Autodesk Fusion 360 part; units mm, degrees
sketch "Sketch1" plane through (0, 12, 0) normal (0, -1, 0) x (1, 0, 0)
  line L0 (-41.8393, 72.4678) -> (-83.6786, 0)
  line L1 (-83.6786, 0) -> (-41.8393, -72.4678)
  line L2 (-41.8393, -72.4678) -> (41.8393, -72.4678)
  line L3 (41.8393, -72.4678) -> (83.6786, 0)
  line L4 (83.6786, 0) -> (41.8393, 72.4678)
  line L5 (41.8393, 72.4678) -> (-41.8393, 72.4678)
  line L6 (-41.8393, 72.4678) -> (41.8393, 72.4678)
  line L7 (41.8393, 72.4678) -> (83.6786, 0)
  line L8 (83.6786, 0) -> (41.8393, -72.4678)
  line L9 (41.8393, -72.4678) -> (-41.8393, -72.4678)
  line L10 (-41.8393, -72.4678) -> (-83.6786, 0)
  line L11 (-83.6786, 0) -> (-41.8393, 72.4678)
  line L12 (82.0621, 0) -> (41.031, -71.0678)
  line L13 (41.031, -71.0678) -> (-41.031, -71.0678)
  line L14 (-41.031, -71.0678) -> (-82.0621, 0)
  line L15 (-82.0621, 0) -> (-41.031, 71.0678)
  line L16 (-41.031, 71.0678) -> (41.031, 71.0678)
  line L17 (41.031, 71.0678) -> (82.0621, 0)
  dimension "d1" = 1.4
sketch "Sketch2" plane through (0, 12, 0) normal (0, 1, 0) x (-1, 0, 0)
  line L0 (-42.4167, 73.4678) -> (42.4167, 73.4678)
  line L1 (42.4167, 73.4678) -> (84.8333, 0)
  line L2 (84.8333, 0) -> (42.4167, -73.4678)
  line L3 (42.4167, -73.4678) -> (-42.4167, -73.4678)
  line L4 (-42.4167, -73.4678) -> (-84.8333, 0)
  line L5 (-84.8333, 0) -> (-42.4167, 73.4678)
  line L6 (-43.5714, 75.4678) -> (-87.1427, 0)
  line L7 (-87.1427, 0) -> (-43.5714, -75.4678)
  line L8 (-43.5714, -75.4678) -> (43.5714, -75.4678)
  line L9 (43.5714, -75.4678) -> (87.1427, 0)
  line L10 (87.1427, 0) -> (43.5714, 75.4678)
  line L11 (43.5714, 75.4678) -> (-43.5714, 75.4678)
  line L12 (-43.5714, 75.4678) -> (43.5714, 75.4678)
  line L13 (87.1427, 0) -> (43.5714, 75.4678)
  line L14 (87.1427, 0) -> (43.5714, -75.4678)
  line L15 (43.5714, -75.4678) -> (-43.5714, -75.4678)
  line L16 (-43.5714, -75.4678) -> (-87.1427, 0)
  line L17 (-87.1427, 0) -> (-43.5714, 75.4678)
sketch "Sketch3" plane through (0, 4, 0) normal (0, 1, 0) x (-1, 0, 0)
  line L0 (-38.9526, -67.4678) -> (-77.9051, 0)
  line L1 (-77.9051, 0) -> (-38.9526, 67.4678)
  line L2 (-38.9526, 67.4678) -> (38.9526, 67.4678)
  line L3 (38.9526, 67.4678) -> (77.9051, 0)
  line L4 (77.9051, 0) -> (38.9526, -67.4678)
  line L5 (38.9526, -67.4678) -> (-38.9526, -67.4678)
  line L6 (-84.8333, 0) -> (-42.4167, -73.4678)
  line L7 (-42.4167, -73.4678) -> (42.4167, -73.4678)
  line L8 (42.4167, -73.4678) -> (84.8333, 0)
  line L9 (84.8333, 0) -> (42.4167, 73.4678)
  line L10 (42.4167, 73.4678) -> (-42.4167, 73.4678)
  line L11 (-42.4167, 73.4678) -> (-84.8333, 0)
  line L12 (42.4167, -73.4678) -> (84.8333, 0)
  line L13 (42.4167, 73.4678) -> (84.8333, 0)
  line L14 (42.4167, 73.4678) -> (-42.4167, 73.4678)
  line L15 (-42.4167, 73.4678) -> (-84.8333, 0)
  line L16 (-84.8333, 0) -> (-42.4167, -73.4678)
  line L17 (-42.4167, -73.4678) -> (42.4167, -73.4678)
  line L18 (-42.4167, 73.4678) -> (-84.8333, 0)
  line L19 (-41.8393, -72.4678) -> (41.8393, -72.4678)
  line L20 (41.8393, -72.4678) -> (83.6786, 0)
  line L21 (41.8393, 72.4678) -> (83.6786, 0)
  line L22 (41.8393, 72.4678) -> (-41.8393, 72.4678)
  line L23 (-41.8393, 72.4678) -> (-83.6786, 0)
  line L24 (-83.6786, 0) -> (-41.8393, -72.4678)
  line L25 (41.031, 71.0678) -> (-41.031, 71.0678)
  line L26 (-41.031, 71.0678) -> (-82.0621, 0)
  line L27 (-82.0621, 0) -> (-41.031, -71.0678)
  line L28 (-41.031, -71.0678) -> (41.031, -71.0678)
  line L29 (41.031, -71.0678) -> (82.0621, 0)
  line L30 (41.031, 71.0678) -> (82.0621, 0)
  dimension "d2" = -1
  dimension "d3" = -2.4
sketch "Sketch4" plane through (0, 13, 0) normal (0, -1, 0) x (1, 0, 0)
  arc A0 (44.7261, 67.4678) -> (36.0658, 72.4678) centre (36.0658, 62.4678) ccw
  line L0 (44.7261, 67.4678) -> (80.7919, 5)
  arc A1 (80.7919, -5) -> (80.7919, 5) centre (72.1316, 0) ccw
  line L1 (80.7919, -5) -> (44.7261, -67.4678)
  arc A2 (36.0658, -72.4678) -> (44.7261, -67.4678) centre (36.0658, -62.4678) ccw
  line L2 (36.0658, -72.4678) -> (-36.0658, -72.4678)
  arc A3 (-44.7261, -67.4678) -> (-36.0658, -72.4678) centre (-36.0658, -62.4678) ccw
  line L3 (-44.7261, -67.4678) -> (-80.7919, -5)
  arc A4 (-80.7919, 5) -> (-80.7919, -5) centre (-72.1316, 0) ccw
  line L4 (-80.7919, 5) -> (-44.7261, 67.4678)
  arc A5 (-36.0658, 72.4678) -> (-44.7261, 67.4678) centre (-36.0658, 62.4678) ccw
  line L5 (-36.0658, 72.4678) -> (36.0658, 72.4678)
  line L6 (42.4167, 73.4678) -> (-42.4167, 73.4678)
  line L7 (-42.4167, 73.4678) -> (-84.8333, 0)
  line L8 (-84.8333, 0) -> (-42.4167, -73.4678)
  line L9 (-42.4167, -73.4678) -> (42.4167, -73.4678)
  line L10 (42.4167, -73.4678) -> (84.8333, 0)
  line L11 (84.8333, 0) -> (42.4167, 73.4678)
  line L12 (-42.4167, 73.4678) -> (-32.4167, 73.4678)
  line L13 (-42.4167, 73.4678) -> (-47.4167, 64.8076)
  line L14 (-32.4167, 73.4678) -> (-32.4167, 56.1473)
  line L15 (-47.4167, 64.8076) -> (-32.4167, 56.1473)
  dimension "d4" = 10
  dimension "d5" = 0
extrude "Extrude1" add sketch "Sketch2" along normal blind 3 contours L0 L1 L2 L3 L4 L5 | L6 L7 L8 L9 L10 L11 L12 L13 L14 L15 L16 L17
extrude "Extrude2" cut sketch "Sketch3" along normal blind -1 and the other way blind -9 contours L6 L7 L8 L9 L10 L11 L12 L13 L14 L15 L16 L17 L18
move_face "OffsetFaces1" [suppressed]
extrude "Extrude3" cut sketch "Sketch1" against normal blind 2.6 contours L12 L13 L14 L15 L16 L17
fillet "Fillet1" radius 10 6 edges at (-83.6786, 12.5, 0) (-41.8393, 12.5, 72.4678) (41.8393, 12.5, 72.4678) (83.6786, 12.5, 0) (41.8393, 12.5, -72.4678) (-41.8393, 12.5, -72.4678)
fillet "Fillet1" radius 10 6 edges at (-41.031, 13.3, 71.0678) (-82.0621, 13.3, 0) (-41.031, 13.3, -71.0678) (41.031, 13.3, -71.0678) (82.0621, 13.3, 0) (41.031, 13.3, 71.0678)
chamfer "Chamfer1" distance 1 angle 45 18 edges at (63.625, 12, 36.7339) (63.625, 12, -36.7339) (82.1316, 12, 0) (62.759, 12, -36.2339) (41.0658, 12, -71.1281) (0, 12, -72.4678) (-41.0658, 12, -71.1281) (-62.759, 12, -36.2339) (-82.1316, 12, 0) (-62.759, 12, 36.2339) (-41.0658, 12, 71.1281) (0, 12, 72.4678) (41.0658, 12, 71.1281) (62.759, 12, 36.2339) (0, 12, 73.4678) (-63.625, 12, 36.7339) (-63.625, 12, -36.7339) (0, 12, -73.4678)
sketch "Sketch5" plane through (0, 14.6, 0) normal (0, -1, 0) x (1, 0, 0)
  arc A0 (43.9178, 66.0678) -> (35.2575, 71.0678) centre (35.2575, 61.0678) ccw
  line L0 (35.2575, 71.0678) -> (-35.2575, 71.0678)
  arc A1 (-35.2575, 71.0678) -> (-43.9178, 66.0678) centre (-35.2575, 61.0678) ccw
  line L1 (-43.9178, 66.0678) -> (-79.1753, 5)
  arc A2 (-79.1753, 5) -> (-79.1753, -5) centre (-70.515, 0) ccw
  line L2 (-79.1753, -5) -> (-43.9178, -66.0678)
  arc A3 (-43.9178, -66.0678) -> (-35.2575, -71.0678) centre (-35.2575, -61.0678) ccw
  line L3 (-35.2575, -71.0678) -> (35.2575, -71.0678)
  arc A4 (35.2575, -71.0678) -> (43.9178, -66.0678) centre (35.2575, -61.0678) ccw
  line L4 (43.9178, -66.0678) -> (79.1753, -5)
  arc A5 (79.1753, -5) -> (79.1753, 5) centre (70.515, 0) ccw
  line L5 (79.1753, 5) -> (43.9178, 66.0678)
  line L6 (0, 0) -> (-80.515, 0)
  line L7 (-40.2575, 69.7281) -> (0, 0)
  line L8 (40.2575, 69.7281) -> (-40.2575, -69.7281)
  line L9 (40.2575, -69.7281) -> (0, 0)
  line L10 (80.515, 0) -> (0, 0)
extrude "Extrude11" add 1 faces at (2.8868, 14.6, -1.6667) along direction (0, -1, 0) blind 3
extrude "Extrude5" [suppressed]
extrude "Extrude6" [suppressed]
extrude "Extrude7" [suppressed]
extrude "Extrude8" [suppressed]
extrude "Extrude9" [suppressed]
sketch "Sketch6" plane through (0, 12, 0) normal (0, -1, 0) x (1, 0, 0)
  line L0 (-35.2575, 71.0678) -> (35.2575, 71.0678)
  arc A0 (43.9178, 66.0678) -> (35.2575, 71.0678) centre (35.2575, 61.0678) ccw
  line L1 (43.9178, 66.0678) -> (79.1753, 5)
  arc A1 (79.1753, -5) -> (79.1753, 5) centre (70.515, 0) ccw
  line L2 (79.1753, -5) -> (43.9178, -66.0678)
  arc A2 (35.2575, -71.0678) -> (43.9178, -66.0678) centre (35.2575, -61.0678) ccw
  line L3 (35.2575, -71.0678) -> (-35.2575, -71.0678)
  arc A3 (-43.9178, -66.0678) -> (-35.2575, -71.0678) centre (-35.2575, -61.0678) ccw
  line L4 (-43.9178, -66.0678) -> (-79.1753, -5)
  arc A4 (-79.1753, 5) -> (-79.1753, -5) centre (-70.515, 0) ccw
  line L5 (-79.1753, 5) -> (-43.9178, 66.0678)
  line L6 (-43.86, 66.9678) -> (-79.9259, 4.5)
  arc A5 (-79.9259, 4.5) -> (-79.9259, -4.5) centre (-72.1316, 0) ccw
  line L7 (-79.9259, -4.5) -> (-43.86, -66.9678)
  arc A6 (-43.86, -66.9678) -> (-36.0658, -71.4678) centre (-36.0658, -62.4678) ccw
  line L8 (-36.0658, -71.4678) -> (36.0658, -71.4678)
  arc A7 (36.0658, -71.4678) -> (43.86, -66.9678) centre (36.0658, -62.4678) ccw
  line L9 (43.86, -66.9678) -> (79.9259, -4.5)
  arc A8 (79.9259, -4.5) -> (79.9259, 4.5) centre (72.1316, 0) ccw
  line L10 (79.9259, 4.5) -> (43.86, 66.9678)
  arc A9 (43.86, 66.9678) -> (36.0658, 71.4678) centre (36.0658, 62.4678) ccw
  line L11 (36.0658, 71.4678) -> (-36.0658, 71.4678)
  arc A10 (-35.2575, 71.0678) -> (-43.9178, 66.0678) centre (-35.2575, 61.0678) ccw
  arc A11 (-36.0658, 71.4678) -> (-43.86, 66.9678) centre (-36.0658, 62.4678) ccw
  line L12 (-79.1753, 5) -> (-43.9178, 66.0678)
  arc A12 (-35.2575, 71.0678) -> (-43.9178, 66.0678) centre (-35.2575, 61.0678) ccw
  line L13 (-35.2575, 71.0678) -> (35.2575, 71.0678)
  arc A13 (43.9178, 66.0678) -> (35.2575, 71.0678) centre (35.2575, 61.0678) ccw
  line L14 (43.9178, 66.0678) -> (79.1753, 5)
  arc A14 (79.1753, -5) -> (79.1753, 5) centre (70.515, 0) ccw
  line L15 (79.1753, -5) -> (43.9178, -66.0678)
  arc A15 (35.2575, -71.0678) -> (43.9178, -66.0678) centre (35.2575, -61.0678) ccw
  line L16 (35.2575, -71.0678) -> (-35.2575, -71.0678)
  arc A16 (-43.9178, -66.0678) -> (-35.2575, -71.0678) centre (-35.2575, -61.0678) ccw
  line L17 (-43.9178, -66.0678) -> (-79.1753, -5)
  arc A17 (-79.1753, 5) -> (-79.1753, -5) centre (-70.515, 0) ccw
  arc A18 (79.9259, -4.5) -> (79.9259, 4.5) centre (72.1316, 0) ccw
  line L18 (79.9259, 4.5) -> (43.86, 66.9678)
  arc A19 (43.86, 66.9678) -> (36.0658, 71.4678) centre (36.0658, 62.4678) ccw
  line L19 (36.0658, 71.4678) -> (-36.0658, 71.4678)
  arc A20 (-36.0658, 71.4678) -> (-43.86, 66.9678) centre (-36.0658, 62.4678) ccw
  line L20 (-43.86, 66.9678) -> (-79.9259, 4.5)
  arc A21 (-79.9259, 4.5) -> (-79.9259, -4.5) centre (-72.1316, 0) ccw
  line L21 (-79.9259, -4.5) -> (-43.86, -66.9678)
  arc A22 (-43.86, -66.9678) -> (-36.0658, -71.4678) centre (-36.0658, -62.4678) ccw
  line L22 (-36.0658, -71.4678) -> (36.0658, -71.4678)
  arc A23 (36.0658, -71.4678) -> (43.86, -66.9678) centre (36.0658, -62.4678) ccw
  line L23 (43.86, -66.9678) -> (79.9259, -4.5)
  arc A24 (42.8785, 65.4678) -> (35.2575, 69.8678) centre (35.2575, 61.0678) ccw
  line L24 (-35.2575, 69.8678) -> (35.2575, 69.8678)
  arc A25 (-35.2575, 69.8678) -> (-42.8785, 65.4678) centre (-35.2575, 61.0678) ccw
  line L25 (-78.1361, 4.4) -> (-42.8785, 65.4678)
  arc A26 (-78.1361, 4.4) -> (-78.1361, -4.4) centre (-70.515, 0) ccw
  line L26 (-42.8785, -65.4678) -> (-78.1361, -4.4)
  arc A27 (-42.8785, -65.4678) -> (-35.2575, -69.8678) centre (-35.2575, -61.0678) ccw
  line L27 (35.2575, -69.8678) -> (-35.2575, -69.8678)
  arc A28 (35.2575, -69.8678) -> (42.8785, -65.4678) centre (35.2575, -61.0678) ccw
  line L28 (78.1361, -4.4) -> (42.8785, -65.4678)
  arc A29 (78.1361, -4.4) -> (78.1361, 4.4) centre (70.515, 0) ccw
  line L29 (42.8785, 65.4678) -> (78.1361, 4.4)
  arc A30 (-35.2575, 70.0678) -> (-43.0518, 65.5678) centre (-35.2575, 61.0678) ccw
  line L30 (-78.3093, 4.5) -> (-43.0518, 65.5678)
  arc A31 (-78.3093, 4.5) -> (-78.3093, -4.5) centre (-70.515, 0) ccw
  line L31 (-43.0518, -65.5678) -> (-78.3093, -4.5)
  arc A32 (-43.0518, -65.5678) -> (-35.2575, -70.0678) centre (-35.2575, -61.0678) ccw
  line L32 (35.2575, -70.0678) -> (-35.2575, -70.0678)
  arc A33 (35.2575, -70.0678) -> (43.0518, -65.5678) centre (35.2575, -61.0678) ccw
  line L33 (78.3093, -4.5) -> (43.0518, -65.5678)
  arc A34 (78.3093, -4.5) -> (78.3093, 4.5) centre (70.515, 0) ccw
  line L34 (43.0518, 65.5678) -> (78.3093, 4.5)
  arc A35 (43.0518, 65.5678) -> (35.2575, 70.0678) centre (35.2575, 61.0678) ccw
  line L35 (-35.2575, 70.0678) -> (35.2575, 70.0678)
  dimension "d16" = 1.2
  dimension "d17" = 1
extrude "Extrude10" [suppressed]
extrude "Extrude4" [suppressed]
chamfer "Chamfer2" [suppressed]
equation "d5 = d154"
The listing builds one solid part. Answer for the finished solid, in the listing's coordinates (mm). A direction names the side the tool comes from. Give positions to 0.01 mm unless a question says otherwise; leave off trailing zeros. Loops run counter-clockwise (first coordinate to the right, second up) from the corner with the lowest first, then second, coordinate; pieces in that order, holes last. Notation, with made-up numbers: M -28,-35 L 5,-35 A25 ccw 5,-2 Z; hole C 71,58 d10. An arc over 180 degrees is marked long. One line per item, written item: value.
Q1. A cutting plane is placed at A-A on y = 14. Determine the outline of the cut face in (x, z).
Working result:
outline: M -87.14,0 L -43.57,-75.47 L 43.57,-75.47 L 87.14,0 L 43.57,75.47 L -43.57,75.47 Z
Q2. For faces 4 (the face through (40.194, 11.803, 69.764)), 5 (the face through (-40.194, 11.803, -69.764)), 6 (the face through (40.32, 11.8, -69.69)), 7 (the face through (40.77, 12.28, -70.47)), determine the directions among +Z, -Z, +X, -X, +Y, -Y from which every point of the face is accessible in a straight line to the end or side of a thin tool.
Working result:
face 4: +Z, +X, -Y
face 5: -Z, -X, -Y
face 6: -Z, +X, -Y
face 7: -Y
Q3. Determine the mould class of faces 1 (the face through (40.649, 12.285, 70.543)), 2 (the face through (1, 15, 1)), 3 (the face through (65.052, 13.479, 38.262)) for opening direction Z: +Z half, -Z half, draft (parallel to the pull), parting line (faces both ways), or undercut.
Working result:
face 1: undercut
face 2: draft
face 3: +Z half
Q4. Find the intervals of material crossed by line 1 (X direction, y = 12.8, z = 47); line 2 (Z direction, x = -75, y = 12.05); line 3 (Z direction, x = -44.5, y = 12.7), in increasing order. Write a range as from..to.
Working result:
line 1: x = -60.01..-57.93, -56.31..56.31, 57.93..60.01
line 2: z = -21.03..-18.93, -13.13..13.13, 18.93..21.03
line 3: z = -73.86..-70.46, -67.26..67.26, 70.46..73.86
Q5. A flat-ended cylindrical pin translates along its axis: P1, Ø2, axis at y = 13, z = -53.5, coming from the -X side. Find the tip coordinate at first contact, or state that the pin passes through.
Working result:
P1: stops at x = -56.83
